Can you work these out from the model? Positions are in its coordinate system, mm. A direction names the side the tool comes from. Give positions to 0.01 mm unless a question says otherwise; leave off trailing zeros. Order: outer loops, then holes, each group sorted by start corner. A loop starts at its lowest first (then second) coordinate and runs counter-clockwise, first axis right, second up. Notation, with made-up numbers: (72.5, 82) - (85.5, 82) arc R34 cw to (85.5, 118) - close; hole circle Ø6 at (-39, 16.25). An arc over 180 degrees is marked (long way). One line per question, with ' | ' between items.
```python
from build123d import *

# Parameters (mm, degrees)
EXTRUDE_1_DEPTH     = 58.89737674
EXTRUDE_START       = 38.399597665
EXTRUDE_2_DEPTH     = 38.399597665
EXTRUDE_3_REACH     = 66.893
SKETCH_3_W          = 44.2
SKETCH_3_H          = 3
EXTRUDE_4_REACH     = 66.893
SKETCH_4_W          = 44.2
SKETCH_4_H          = 3
CUT_EXTRUDE_START   = -77.29697691
CUT_EXTRUDE_1_DEPTH = 77.29697691
SKETCH_6_W          = 16.122631446
SKETCH_6_H          = 4.394864928
CUT_EXTRUDE_2_DEPTH = 3
EXTRUDE_START_2     = 15
EXTRUDE_5_DEPTH     = 15


with BuildPart() as part:
    # 草图1 → 凸台-拉伸1 (new body)
    with BuildSketch(Plane(origin=(0, 0, 0), x_dir=(1, 0, 0), z_dir=(0, 1, 0))):
        with BuildLine():
            Line((21.346642729, -10.719560241), (16.852020459, -16.362765964))
            ThreePointArc((16.852020459, -16.362765964), (15.807857901, -17.196247295), (14.505374257, -17.493741725))
            Line((14.505374257, -17.493741725), (-14.505381202, -17.493741725))
            ThreePointArc((-14.505381202, -17.493741725), (-15.807864846, -17.196247295), (-16.852027404, -16.362765964))
            Line((-16.852027404, -16.362765964), (-21.346649674, -10.719560241))
            ThreePointArc((-21.346649674, -10.719560241), (-21.831958504, -9.840501001), (-22.000003473, -8.850536003))
            Line((-22.000003473, -8.850536003), (-23.000003473, -8.850536003))
            ThreePointArc((-23.000003473, -8.850536003), (-23.707110254, -8.557642784), (-24.000003473, -7.850536003))
            Line((-24.000003473, -7.850536003), (-24.000003473, -1.349569462))
            ThreePointArc((-24.000003473, -1.349569462), (-23.707110254, -0.642462681), (-23.000003473, -0.349569462))
            Line((-23.000003473, -0.349569462), (-22.100003473, -0.349569462))
            Line((-22.100003473, -0.349569462), (-22.100003473, -4.600052733))
            Line((-22.100003473, -4.600052733), (-22.000003473, -4.600052733))
            Line((-22.000003473, -4.600052733), (-20.000003473, -4.600052733))
            Line((-20.000003473, -4.600052733), (-20.000003473, -9.200105465))
            Line((-20.000003473, -9.200105465), (-14.987335304, -15.493741725))
            Line((-14.987335304, -15.493741725), (14.987328359, -15.493741725))
            Line((14.987328359, -15.493741725), (19.999996527, -9.200105465))
            Line((19.999996527, -9.200105465), (19.999996527, -4.600052733))
            Line((19.999996527, -4.600052733), (21.999996527, -4.600052733))
            Line((21.999996527, -4.600052733), (22.099996527, -4.600052733))
            Line((22.099996527, -4.600052733), (22.099996527, -0.349569462))
            Line((22.099996527, -0.349569462), (22.999996527, -0.349569462))
            ThreePointArc((22.999996527, -0.349569462), (23.707103309, -0.642462681), (23.999996527, -1.349569462))
            Line((23.999996527, -1.349569462), (23.999996527, -7.850536003))
            ThreePointArc((23.999996527, -7.850536003), (23.707103309, -8.557642784), (22.999996527, -8.850536003))
            Line((22.999996527, -8.850536003), (21.999996527, -8.850536003))
            ThreePointArc((21.999996527, -8.850536003), (21.831951559, -9.840501001), (21.346642729, -10.719560241))
        make_face()
    extrude(amount=EXTRUDE_1_DEPTH)

    # 草图2 → 凸台-拉伸2 (add)
    with BuildSketch(Plane.XZ.offset(EXTRUDE_START)):
        with BuildLine():
            Line((22.999996527, 8.850536003), (21.999996527, 8.850536003))
            ThreePointArc((21.999996527, 8.850536003), (21.831951559, 9.840501001), (21.346642729, 10.719560241))
            Line((21.346642729, 10.719560241), (16.852020459, 16.362765964))
            ThreePointArc((16.852020459, 16.362765964), (15.807857901, 17.196247295), (14.505374257, 17.493741725))
            Line((14.505374257, 17.493741725), (-14.505381202, 17.493741725))
            ThreePointArc((-14.505381202, 17.493741725), (-15.807864846, 17.196247295), (-16.852027404, 16.362765964))
            Line((-16.852027404, 16.362765964), (-21.346649674, 10.719560241))
            ThreePointArc((-21.346649674, 10.719560241), (-21.831958504, 9.840501001), (-22.000003473, 8.850536003))
            Line((-22.000003473, 8.850536003), (-23.000003473, 8.850536003))
            ThreePointArc((-23.000003473, 8.850536003), (-23.707110254, 8.557642784), (-24.000003473, 7.850536003))
            Line((-24.000003473, 7.850536003), (-24.000003473, 1.349569462))
            ThreePointArc((-24.000003473, 1.349569462), (-23.707110254, 0.642462681), (-23.000003473, 0.349569462))
            Line((-23.000003473, 0.349569462), (-22.100003473, 0.349569462))
            Line((-22.100003473, 0.349569462), (-22.100003473, 4.600052733))
            Line((-22.100003473, 4.600052733), (-20.000003473, 4.600052733))
            Line((-20.000003473, 4.600052733), (-20.000003473, 9.200105465))
            Line((-20.000003473, 9.200105465), (-14.987335304, 15.493741725))
            Line((-14.987335304, 15.493741725), (14.987328359, 15.493741725))
            Line((14.987328359, 15.493741725), (19.999996527, 9.200105465))
            Line((19.999996527, 9.200105465), (19.999996527, 4.600052733))
            Line((19.999996527, 4.600052733), (22.099996527, 4.600052733))
            Line((22.099996527, 4.600052733), (22.099996527, 0.349569462))
            Line((22.099996527, 0.349569462), (22.999996527, 0.349569462))
            ThreePointArc((22.999996527, 0.349569462), (23.707103309, 0.642462681), (23.999996527, 1.349569462))
            Line((23.999996527, 1.349569462), (23.999996527, 7.850536003))
            ThreePointArc((23.999996527, 7.850536003), (23.707103309, 8.557642784), (22.999996527, 8.850536003))
        make_face()
    extrude(amount=-EXTRUDE_2_DEPTH)

    # 凸台-拉伸3: up to this face of the body (flat: up to its plane)
    extrude_3_end = Plane(part.part.faces().sort_by_distance((-3.473e-06, 10.248889538, 17.493741725))[0])
    # 草图3 → 凸台-拉伸3 (add, up to the picked face)
    with BuildSketch(Plane(origin=(0, 0, 4.600052733), x_dir=(-1, 0, 0), z_dir=(0, 0, -1)), mode=Mode.PRIVATE) as extrude_3_sk1:
        with Locations((3.473e-06, -36.899597665)):
            Rectangle(SKETCH_3_W, SKETCH_3_H)
    extrude_3_tool1 = split(extrude(extrude_3_sk1.sketch, amount=-EXTRUDE_3_REACH, mode=Mode.PRIVATE), bisect_by=extrude_3_end, keep=Keep.BOTH, mode=Mode.PRIVATE)
    add(extrude_3_tool1.solids().sort_by(Axis((-3e-06, -36.899598, 4.600053), (0, 0, 1)))[0])

    # 凸台-拉伸4: up to this face of the body (flat: up to its plane)
    extrude_4_end = Plane(part.part.faces().sort_by_distance((-3.473e-06, 9.499837909, 17.493741725))[0])
    # 草图4 → 凸台-拉伸4 (add, up to the picked face)
    with BuildSketch(Plane(origin=(0, 0, 4.600052733), x_dir=(-1, 0, 0), z_dir=(0, 0, -1)), mode=Mode.PRIVATE) as extrude_4_sk1:
        with Locations((3.473e-06, 37.397379245)):
            Rectangle(SKETCH_4_W, SKETCH_4_H)
    extrude_4_tool1 = split(extrude(extrude_4_sk1.sketch, amount=-EXTRUDE_4_REACH, mode=Mode.PRIVATE), bisect_by=extrude_4_end, keep=Keep.BOTH, mode=Mode.PRIVATE)
    add(extrude_4_tool1.solids().sort_by(Axis((-3e-06, 37.397379, 4.600053), (0, 0, 1)))[0])

    # 草图5 → 切除-拉伸1 (cut)
    with BuildSketch(Plane(origin=(0, 38.897379245, 0), x_dir=(1, 0, 0), z_dir=(0, 1, 0)).offset(CUT_EXTRUDE_START)):
        with BuildLine():
            Line((-22.100003473, -8.850536003), (-22.100003473, -17.493741725))
            Line((-22.100003473, -17.493741725), (-14.505381202, -17.493741725))
            ThreePointArc((-14.505381202, -17.493741725), (-15.807864846, -17.196247295), (-16.852027404, -16.362765964))
            Line((-16.852027404, -16.362765964), (-21.346649674, -10.719560241))
            ThreePointArc((-21.346649674, -10.719560241), (-21.831958504, -9.840501001), (-22.000003473, -8.850536003))
            Line((-22.000003473, -8.850536003), (-22.100003473, -8.850536003))
        make_face()
        with BuildLine():
            Line((14.505374257, -17.493741725), (22.099996527, -17.493741725))
            Line((22.099996527, -17.493741725), (22.099996527, -8.850536003))
            Line((22.099996527, -8.850536003), (21.999996527, -8.850536003))
            ThreePointArc((21.999996527, -8.850536003), (21.831951559, -9.840501001), (21.346642729, -10.719560241))
            Line((21.346642729, -10.719560241), (16.852020459, -16.362765964))
            ThreePointArc((16.852020459, -16.362765964), (15.807857901, -17.196247295), (14.505374257, -17.493741725))
        make_face()
    extrude(amount=CUT_EXTRUDE_1_DEPTH, mode=Mode.SUBTRACT)

    # 草图6 → 切除-拉伸2 (cut)
    with BuildSketch(Plane(origin=(0, 38.897379245, 0), x_dir=(1, 0, 0), z_dir=(0, 1, 0))):
        with Locations((0, -9.597483264)):
            Rectangle(SKETCH_6_W, SKETCH_6_H)
    extrude(amount=-CUT_EXTRUDE_2_DEPTH, mode=Mode.SUBTRACT)

    # 草图7 → 凸台-拉伸5 (add)
    with BuildSketch(Plane(origin=(0, -38.399597665, 0), x_dir=(-1, 0, 0), z_dir=(0, -1, 0)).offset(EXTRUDE_START_2)):
        with BuildLine():
            Line((20.000003473, -4.600052733), (20.000003473, -9.200105465))
            Line((20.000003473, -9.200105465), (14.987335304, -15.493741725))
            Line((14.987335304, -15.493741725), (-14.987328359, -15.493741725))
            Line((-14.987328359, -15.493741725), (-19.999996527, -9.200105465))
            Line((-19.999996527, -9.200105465), (-19.999996527, -4.600052733))
            Line((-19.999996527, -4.600052733), (-21.999996527, -4.600052733))
            Line((-21.999996527, -4.600052733), (-22.099996527, -4.600052733))
            Line((-22.099996527, -4.600052733), (-22.099996527, -0.349569462))
            Line((-22.099996527, -0.349569462), (-22.999996527, -0.349569462))
            ThreePointArc((-22.999996527, -0.349569462), (-23.707103309, -0.642462681), (-23.999996527, -1.349569462))
            Line((-23.999996527, -1.349569462), (-23.999996527, -7.850536003))
            ThreePointArc((-23.999996527, -7.850536003), (-23.707103309, -8.557642784), (-22.999996527, -8.850536003))
            Line((-22.999996527, -8.850536003), (-21.999996527, -8.850536003))
            ThreePointArc((-21.999996527, -8.850536003), (-21.831951559, -9.840501001), (-21.346642729, -10.719560241))
            Line((-21.346642729, -10.719560241), (-16.852020459, -16.362765964))
            ThreePointArc((-16.852020459, -16.362765964), (-15.807857901, -17.196247295), (-14.505374257, -17.493741725))
            Line((-14.505374257, -17.493741725), (14.505381202, -17.493741725))
            ThreePointArc((14.505381202, -17.493741725), (15.807864846, -17.196247295), (16.852027404, -16.362765964))
            Line((16.852027404, -16.362765964), (21.346649674, -10.719560241))
            ThreePointArc((21.346649674, -10.719560241), (21.831958504, -9.840501001), (22.000003473, -8.850536003))
            Line((22.000003473, -8.850536003), (23.000003473, -8.850536003))
            ThreePointArc((23.000003473, -8.850536003), (23.707110254, -8.557642784), (24.000003473, -7.850536003))
            Line((24.000003473, -7.850536003), (24.000003473, -1.349569462))
            ThreePointArc((24.000003473, -1.349569462), (23.707110254, -0.642462681), (23.000003473, -0.349569462))
            Line((23.000003473, -0.349569462), (22.100003473, -0.349569462))
            Line((22.100003473, -0.349569462), (22.100003473, -4.600052733))
            Line((22.100003473, -4.600052733), (22.000003473, -4.600052733))
            Line((22.000003473, -4.600052733), (20.000003473, -4.600052733))
        make_face()
    extrude(amount=-EXTRUDE_5_DEPTH)

    # 草图8 → 切除-旋转1 (revolve, cut)
    with BuildSketch(Plane(origin=(0, 0, 0), x_dir=(0, 0, -1), z_dir=(1, 0, 0))):
        Polygon((-9.89924439, -38.299597665), (-20.291549236, -44.299597665), (-20.291549236, -55.801852499), (11.09144377, -55.801852499), (11.09144377, -44.299597665), (0.699138925, -38.299597665), align=None)
    revolve(axis=Axis((0, -108.399597665, 9.89924439), (0, 0, -1)), mode=Mode.SUBTRACT)


solid = part.part
```
(1) If I drill on line 1 (Y direction, x = 15, z = 7.25); line 2 (X direction, y = -37.5, z = 3.75); line 3 (X direction, y = 9, z = 6.75), over which ranges is the centre line in solid material (lowest first)?
Answer below:
line 1: -38.4 to -35.4, 35.9 to 38.9 | line 2: -24 to -22.1, 22.1 to 24 | line 3: -24 to -20, 20 to 24
(2) Imagine slicing it at B-B (y = -36.5). List the corners of the cut face in (x, z) for me.
Answer below:
outline: (-24, 1.35) arc R1 ccw to (-23, 0.35) - (-22.1, 0.35) - (-22.1, 4.6) - (22.1, 4.6) - (22.1, 0.35) - (23, 0.35) arc R1 ccw to (24, 1.35) - (24, 7.85) arc R1 ccw to (23, 8.85) - (22, 8.85) arc R3 ccw to (21.35, 10.72) - (16.85, 16.36) arc R3 ccw to (14.51, 17.49) - (-14.51, 17.49) arc R3 ccw to (-16.85, 16.36) - (-21.35, 10.72) arc R3 ccw to (-22, 8.85) - (-23, 8.85) arc R1 ccw to (-24, 7.85) - close
(3) Imagine slicing it at C-C (z = 13). List the corners of the cut face in (x, y) for me, and give its area (3 significant figures).
Answer below:
outline: (-19.53, -42.94) arc R68.31 cw to (-16.97, -42.23) - (-16.97, -38.4) - (16.97, -38.4) - (16.97, -42.23) arc R68.31 cw to (19.53, -42.94) - (19.53, 58.9) - (16.97, 58.9) - (16.97, 38.9) - (-16.97, 38.9) - (-16.97, 58.9) - (-19.53, 58.9) - close; hole (-16.97, -35.4) - (16.97, -35.4) - (16.97, 35.9) - (-16.97, 35.9) - close | area: 723 mm^2
(4) On a 3-axis mill with a long thin cutter (end or side, diameter ignored), from which of +Z, -Z, +X, -X, +Y, -Y can I reach the whole of each face in a straight line? I mean faces 4 (the face through (-20, -40, 7)), 5 (the face through (-17.53, 48.76, 12.3)), 6 (the face through (0, 37, 7.4)). Say none if no direction works.
Answer below:
face 4: -Z, -Y | face 5: -Z, +Y | face 6: +Y
(5) Imagine slicing it at A-A (z = 6.25). List the corners of the cut face in (x, y) for me, and give its area (3 significant figures).
Answer below:
outline: (-24, -42.54) arc R70.1 cw to (-20, -41.21) - (-20, -38.4) - (-3.74, -38.4) arc R70.1 cw to (3.74, -38.4) - (20, -38.4) - (20, -41.21) arc R70.1 cw to (24, -42.54) - (24, 58.9) - (20, 58.9) - (20, 38.9) - (-20, 38.9) - (-20, 58.9) - (-24, 58.9) - close; hole (-20, -35.4) - (20, -35.4) - (20, 35.9) - (-20, 35.9) - close | area: 1,050 mm^2
(6) If we mould it in two halves opening along Y, with no side actions, what happens to faces 1 (the face through (0, 7, 17.494)), 2 (the face through (0, 35.897, 12)), 3 (the face through (0, 38.897, 12))? For each: released by +Y, released by -Y, zero draft, split by the parting line, or undercut.
Answer below:
face 1: zero draft | face 2: undercut | face 3: released by +Y
(7) Will these pins go through, and if not, where does the flat tip stop? pin 1 (2.5 mm diameter, centred on x = -5.5, y = -40, fed in from -Z); pin 2 (8 mm diameter, centred on x = 12, z = 11, fed in from +Y); pin 3 (4 mm diameter, centred on x = -11, z = 9, fed in from -Y).
Answer below:
pin 1: z = 15.49 | pin 2: y = 38.9 | pin 3: y = -38.4
